from build123d import *

# Parameters (mm, degrees)
SKETCH1_W           = 12.4
SKETCH1_H           = 58
BOSS_EXTRUDE1_DEPTH = 5
CUT_EXTRUDE1_DEPTH  = 3
SKETCH4_R           = 4
CUT_EXTRUDE2_DEPTH  = 5


with BuildPart() as part:
    # Sketch1 → Boss-Extrude1 (new body)
    with BuildSketch(Plane.XY):
        Rectangle(SKETCH1_W, SKETCH1_H)
    extrude(amount=-BOSS_EXTRUDE1_DEPTH)

    # Sketch2 → Cut-Extrude1 (cut)
    with BuildSketch(Plane.XY):
        Polygon((-3.613807992, 0), (-2.3482015, 18.253803872), (0, 18.387804485), (2.3482015, 18.253803872), (3.613807992, 0), (2.3482015, -18.253803872), (0, -18.387804485), (-2.3482015, -18.253803872), align=None)
    extrude(amount=-CUT_EXTRUDE1_DEPTH, mode=Mode.SUBTRACT)

    # Sketch4 → Cut-Extrude2 (cut)
    with BuildSketch(Plane.XY):
        Circle(SKETCH4_R)
    extrude(amount=-CUT_EXTRUDE2_DEPTH, mode=Mode.SUBTRACT)


solid = part.part
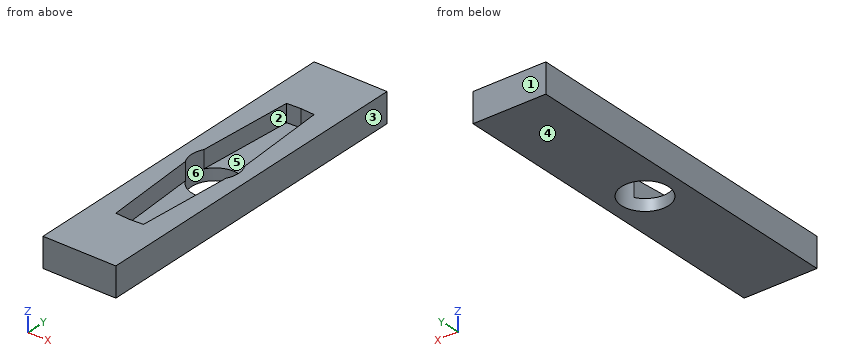
Read the model definition and answer for the solid it produces. Units are mm, in the model's axes. Face numbers are marked on the shaded views. A direction names the side the tool comes from. Round coordinates to 2 decimals unless told otherwise and drop trailing zeros. Loops run counter-clockwise (first coordinate to the right, second up) from the corner with the lowest first, then second, coordinate; pieces in that order, holes last.
Q1. Section C-C on x = 3 is taken. Write down the section's boundary in (y, z), and give its area (3 significant figures).
Q2. Determine the mould class of the marked faces 3, 4, 5 and 6 for opening direction X: released by +X, released by -X, zero draft, split by the parting line, or undercut.
Q3. Section A-A on y = 0 is taken. Write down the section's boundary in (x, z), and give its area (3 significant figures).
Q4. Each of these flat-tipped pins is pushed along its axis until it touches: pin 1 (2 mm diameter, centred on x = -0.5, y = -11, fed in from +Z); pin 2 (6.5 mm diameter, centred on x = 0, y = 0, fed in from -Z); pin 3 (4 mm diameter, centred on x = 3, y = 12.5, fed in from +Z). Where does it stop, or does it pass through?
Q5. Section B-B on z = -0.55 is taken. Write down the section's boundary in (x, y).
Q6. Section D-D on y = -15.5 is taken. Write down the section's boundary in (x, z).
Q7. Consider probe 1 along Y at (x, z) = (0, -2); probe 2 along Y at (x, z) = (-2.25, -0.7); probe 3 along X at (y, z) = (0, -3.7). Determine where each line is inside the solid, lowest interval first.
Q8. Which of the six approach directions +Z, -Z, +X, -X, +Y, -Y give full straight-line access (tool end or side, diameter ignored) to the marked faces 1 and 2?
Output:
1. outline: (-29, -5) - (-2.65, -5) - (-2.65, -3) - (-8.85, -3) - (-8.85, 0) - (-29, 0) - close; (2.65, -5) - (29, -5) - (29, 0) - (8.85, 0) - (8.85, -3) - (2.65, -3) - close
1. area: 226 mm2
2. face 3: released by +X
2. face 4: zero draft
2. face 5: undercut
2. face 6: undercut
3. outline: (-6.2, -5) - (-4, -5) - (-4, 0) - (-6.2, 0) - close; (4, -5) - (6.2, -5) - (6.2, 0) - (4, 0) - close
3. area: 22.0 mm2
4. pin 1: stops at z = -3
4. pin 2: passes through
4. pin 3: stops at z = 0
5. outline: (-6.2, -29) - (6.2, -29) - (6.2, 29) - (-6.2, 29) - close; hole (-3.48, -1.98) - (-2.35, -18.25) - (0, -18.39) - (2.35, -18.25) - (3.48, -1.98) arc R4 ccw to (3.48, 1.98) - (2.35, 18.25) - (0, 18.39) - (-2.35, 18.25) - (-3.48, 1.98) arc R4 ccw to start
6. outline: (-6.2, -5) - (6.2, -5) - (6.2, 0) - (2.54, 0) - (2.54, -3) - (-2.54, -3) - (-2.54, 0) - (-6.2, 0) - close
7. probe 1: y = -29 to -18.39, 18.39 to 29
7. probe 2: y = -29 to -18.26, 18.26 to 29
7. probe 3: x = -6.2 to -4, 4 to 6.2
8. face 1: +Z, -Z, +X, -X, +Y
8. face 2: +Z
